Design review of the part shown in the three views and the two pictorial views. Dimensions are in mm from the part's minimum x, y and z. A direction names the side the tool comes from. Coordinates: 2 decimals unless noted, no trailing zeros. Write each loop counter-clockwise with the first axis right and the second up, starting at its lowest first coordinate (ties: lowest second). Pieces come first, ordered by that corner, then holes.
Q1. For L1, parallel to Z at x = 16.51, y = 2.2; L2, parallel to Z at x = 20.5, y = 1.5; L3, parallel to Z at x = 21.5, y = 3, list the stretches that pass through material, from the lowest coordinate up.
Q2. Take a section at D-D, the plane x = 16.51. Write out the cut boundary in (y, z), plus the area to 3 significant figures.
Q3. The part is to be moulded in two halves that separate along Y. For the marked faces 1, 2 and 3, say which applies: released by +Y, released by -Y, zero draft, split by the parting line, or undercut.
Q4. Take a section at B-B, the plane x = 21.5. Write out the cut boundary in (y, z), plus the area to 3 significant figures.
Q5. Take a section at C-C, the plane y = 6.5. Write out the cut boundary in (x, z).
Q6. For pin 1 Ø1.4 at (x, z) = (21.082, 16.256) entering from +Y; pin 2 Ø6 at (x, z) = (20, 12.5) entering from +Y; pin 3 Ø1.5 at (x, y) = (16.5, 5) entering from +Z, all flat-tipped, find the tip position at first contact; note any pin that passes through.
Q7. For the marked faces 4 and 5, list the 3-axis set-ups (+Z, -Z, +X, -X, +Y, -Y) from which the entire face can be reached by the end or side of a thin tool; tool diameter is ignored.
Q8. Take a section at A-A, the plane z = 12.7. Write out the cut boundary in (x, y), plus the area to 3 significant figures.
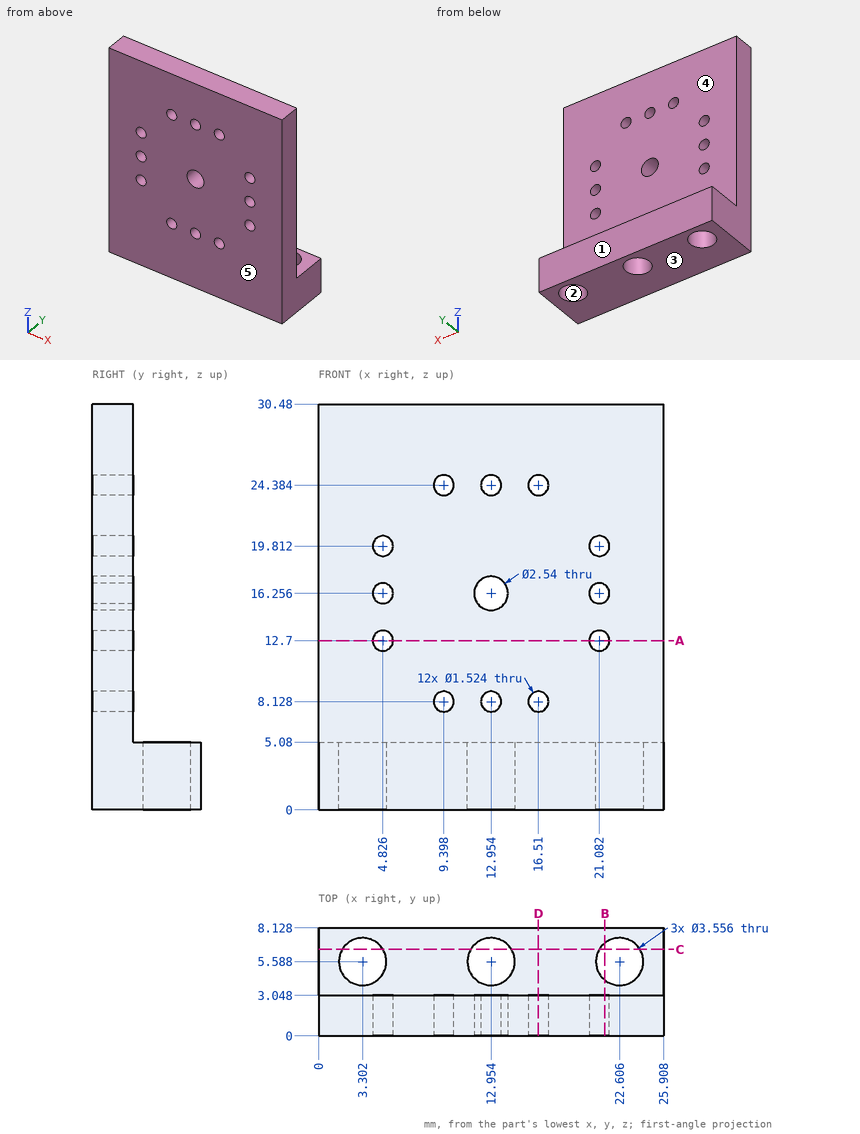
Responses:
1. L1: z = 0 to 7.37, 8.89 to 23.62, 25.15 to 30.48
1. L2: z = 0 to 12.21, 13.19 to 15.76, 16.75 to 19.32, 20.3 to 30.48
1. L3: z = 0 to 12.06, 13.34 to 15.62, 16.89 to 19.17, 20.45 to 30.48
2. outline: (0, 0) - (8.13, 0) - (8.13, 5.08) - (3.05, 5.08) - (3.05, 7.37) - (0, 7.37) - close; (0, 8.89) - (3.05, 8.89) - (3.05, 23.62) - (0, 23.62) - close; (0, 25.15) - (3.05, 25.15) - (3.05, 30.48) - (0, 30.48) - close
2. area: 109 mm2
3. face 1: released by +Y
3. face 2: undercut
3. face 3: zero draft
4. outline: (0, 0) - (4.2, 0) - (4.2, 5.08) - (3.05, 5.08) - (3.05, 12.06) - (0, 12.06) - close; (0, 13.34) - (3.05, 13.34) - (3.05, 15.62) - (0, 15.62) - close; (0, 16.89) - (3.05, 16.89) - (3.05, 19.17) - (0, 19.17) - close; (0, 20.45) - (3.05, 20.45) - (3.05, 30.48) - (0, 30.48) - close; (6.98, 0) - (8.13, 0) - (8.13, 5.08) - (6.98, 5.08) - close
4. area: 92.9 mm2
5. outline: (0, 0) - (1.78, 0) - (1.78, 5.08) - (0, 5.08) - close; (4.83, 0) - (11.43, 0) - (11.43, 5.08) - (4.83, 5.08) - close; (14.48, 0) - (21.08, 0) - (21.08, 5.08) - (14.48, 5.08) - close; (24.13, 0) - (25.91, 0) - (25.91, 5.08) - (24.13, 5.08) - close
6. pin 1: passes through
6. pin 2: stops at y = 3.05
6. pin 3: stops at z = 5.08
7. face 4: +Z, +X, -X, +Y
7. face 5: +Z, -Z, +X, -X, -Y
8. outline: (0, 0) - (4.06, 0) - (4.06, 3.05) - (0, 3.05) - close; (5.59, 0) - (20.32, 0) - (20.32, 3.05) - (5.59, 3.05) - close; (21.84, 0) - (25.91, 0) - (25.91, 3.05) - (21.84, 3.05) - close
8. area: 69.7 mm2
